from build123d import *

# Parameters (mm, degrees)
F0_W     = 51.054
F0_H     = 6.604
F0_W_2   = 4.7625
F0_H_2   = 50.8
F0_W_3   = 50.8
F0_H_3   = 4.7625
F1_DEPTH = 4.7625


with BuildPart() as f1:
    # F0 (on Front) → F1 (new body)
    with BuildSketch(Plane.XZ):
        Polygon((-127, 76.2), (-177.8, 76.2), (-177.8, -25.4), (-177.8, -76.2), (177.8, -76.2), (177.8, -25.4), (177.8, 76.2), (127, 76.2), (76.2, 76.2), (25.4, 76.2), (-25.4, 76.2), (-76.2, 76.2), align=None)
        with Locations((-101.6, 15.875)):
            Rectangle(F0_W, F0_H, mode=Mode.SUBTRACT)
        with Locations((0, 15.875)):
            Rectangle(F0_W, F0_H, mode=Mode.SUBTRACT)
        with Locations((101.6, 15.875)):
            Rectangle(F0_W, F0_H, mode=Mode.SUBTRACT)
        with Locations((180.18125, -50.8)):
            Rectangle(F0_W_2, F0_H_2)
        with Locations((-180.18125, -50.8)):
            Rectangle(F0_W_2, F0_H_2)
        with Locations((-101.6, 78.58125)):
            Rectangle(F0_W_3, F0_H_3)
        with Locations((0, 78.58125)):
            Rectangle(F0_W_3, F0_H_3)
        with Locations((101.6, 78.58125)):
            Rectangle(F0_W_3, F0_H_3)
    extrude(amount=F1_DEPTH)


solid = f1.part
The listing builds one solid part. Answer for the finished solid, in the listing's coordinates (mm). Round coordinates to 2 decimals unless told otherwise and drop trailing zeros. Order: outer loops, then holes, each group sorted by start corner. A loop starts at its lowest first (then second) coordinate and runs counter-clockwise, first axis right, second up. Notation, with made-up numbers: (-38, 24.5) -> (8, 24.5) arc R34 cw to (8, 63.5) -> close; hole circle Ø9 at (56, 37). An arc over 180 degrees is marked (long way). Put each result on its own line as item: value.
Q1. Section A-A, the plane y = -1.35 is taken. Count the separate pieces of the cut face and the enclosed holes in it, and give its area (3 significant figures).
Results list:
separate pieces: 1
enclosed holes: 3
area: 54,400 mm^2
Q2. Consider line 1 along X through (y, z) = (-0.45, 14); line 2 along Z through (x, y) = (-108, -4); line 3 along X through (y, z) = (-3.95, -17). Determine where each line is inside the solid, lowest interval first.
Results list:
line 1: -177.8 to -127.13, -76.07 to -25.53, 25.53 to 76.07, 127.13 to 177.8
line 2: -76.2 to 12.57, 19.18 to 80.96
line 3: -177.8 to 177.8
Q3. Section C-C, the plane x = -64 is taken. Write down the section's boundary in (y, z).
Results list:
outline: (-4.76, -76.2) -> (0, -76.2) -> (0, 76.2) -> (-4.76, 76.2) -> close
Q4. Section D-D, the plane z = 62 is taken. Write down the section's boundary in (x, y), and give its area (3 significant figures).
Results list:
outline: (-177.8, -4.76) -> (177.8, -4.76) -> (177.8, 0) -> (-177.8, 0) -> close
area: 1,690 mm^2
Q5. Section B-B, the plane x = 10 is taken. Write down the section's boundary in (y, z), and give its area (3 significant figures).
Results list:
outline: (-4.76, -76.2) -> (0, -76.2) -> (0, 12.57) -> (-4.76, 12.57) -> close; (-4.76, 19.18) -> (0, 19.18) -> (0, 80.96) -> (-4.76, 80.96) -> close
area: 717 mm^2
Q6. Each of these flat-tipped pins is pushed along its axis until it touches: P1, Ø2.5, axis at x = -141.5, y = -2.5, coming from the +Z side; P2, Ø1.4, axis at y = -3, z = 32, coming from the -X side; P3, Ø2.5, axis at y = -1.5, z = 17, coming from the +X side. Where does it stop, or does it pass through?
Results list:
P1: z = 76.2
P2: x = -177.8
P3: x = 177.8
